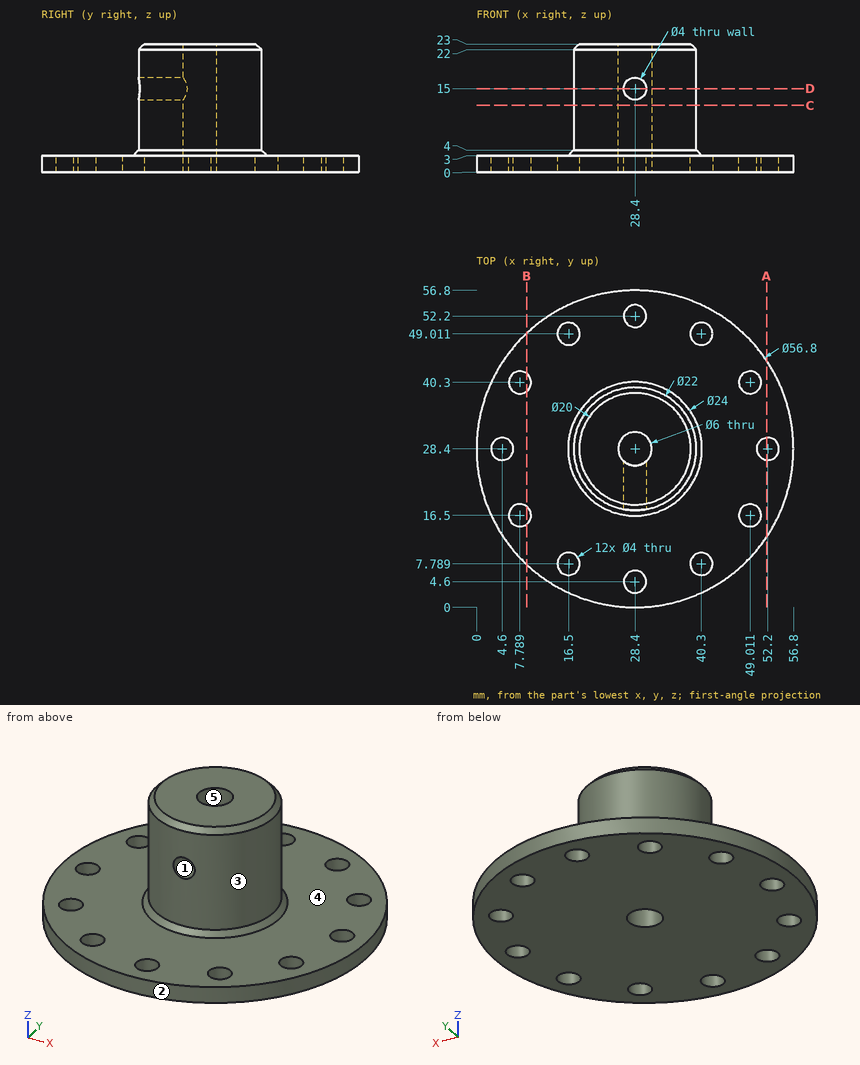
Geometry check sheet. Reference: drawing and pictorial views, mm from the part's lowest x, y, z. A direction names the side the tool comes from. Coordinates: 2 decimals unless noted, no trailing zeros. Write each loop counter-clockwise with the first axis right and the second up, starting at its lowest first coordinate (ties: lowest second). Pieces come first, ordered by that corner, then holes.
Item 1: Cross-section at D-D on z = 15. Record the boundary of the cut face in (x, y).
Numbers:
outline: (26.4, 17.58) - (26.4, 26.16) arc R3 cw (long way) to (30.4, 26.16) - (30.4, 17.58) arc R11 ccw (long way) to start
Item 2: Depth check by flat-ended pin: pin 1 Ø1.5 at (x, y) = (28, 27) entering from +Z; pin 2 Ø4.5 at (x, y) = (7.79, 16.5) entering from +Z; pin 3 Ø8 at (x, z) = (23, 15.5) entering from +Y; pin 4 Ø3.5 at (x, z) = (28.4, 15) entering from -Y. Enter the tip coordinate at first touch or a pass-through.
Numbers:
pin 1: passes through
pin 2: stops at z = 3
pin 3: stops at y = 39.31
pin 4: stops at y = 30.84
Item 3: Scan lines: probe 1 along X at (y, z) = (40.3, 1.2); probe 2 along Z at (x, y) = (20, 7.5). Record each from-to range of solid material in increasing order.
Numbers:
probe 1: x = 2.61 to 5.79, 9.79 to 47.01, 51.01 to 54.19
probe 2: z = 0 to 3
Item 4: Access from +Z, -Z, +X, -X, +Y, -Y to the whole of each face (thin tool, end or side, straight path). Record for the marked faces 1 and 2.
Numbers:
face 1: -Y
face 2: +Z, -Z
Item 5: Mould release check, pull along X, two halves, no side actions. Record for the marked faces 3, 4 and 5: released by +X, released by -X, zero draft, split by the parting line, or undercut.
Numbers:
face 3: split by the parting line
face 4: zero draft
face 5: undercut
Item 6: Cross-section at A-A on x = 52. Record the boundary of the cut face in (y, z).
Numbers:
outline: (12.6, 0) - (26.41, 0) - (26.41, 3) - (12.6, 3) - close; (30.39, 0) - (44.2, 0) - (44.2, 3) - (30.39, 3) - close
Item 7: Cross-section at C-C on z = 12. Record the boundary of the cut face in (x, y), then the cut area to 3 significant figures.
Numbers:
outline: circle Ø22 at (28.4, 28.4); hole circle Ø6 at (28.4, 28.4)
area: 352 mm2
Item 8: Cross-section at B-B on x = 9. Record the boundary of the cut face in (y, z).
Numbers:
outline: (7.66, 0) - (14.91, 0) - (14.91, 3) - (7.66, 3) - close; (18.09, 0) - (38.71, 0) - (38.71, 3) - (18.09, 3) - close; (41.89, 0) - (49.14, 0) - (49.14, 3) - (41.89, 3) - close
